Check sheet for the modelled part. Datum: model origin and axes. Units: mm. Round coordinates to 2 decimals unless told otherwise and drop trailing zeros. Loops run counter-clockwise (first coordinate to the right, second up) from the corner with the lowest first, then second, coordinate; pieces in that order, holes last. Notation, with made-up numbers: (62.5, -1.5) -> (73.5, -1.5) arc R30 ccw to (73.5, 32.5) -> close; hole circle Ø5 at (47.25, -16.5). An arc over 180 degrees is marked (long way). Use one line per item in the form item = value. Start each with the question number.
(1) Draft check along X on faces 1 (the cylindrical face through (74.1, -12.3, 45.4)), 2 (the cylindrical face through (76.7, -12.3, 40.1)), 3 (the flat face through (83, -25, 38)). Enter one of: released by +X, released by -X, zero draft, split by the parting line, or undercut.
(2) Sectioned sample at A-A (z = 40). Record the cut outline in (x, y).
(3) Go/stop test with flat-tipped pins: pin 1 (1 mm diameter, centred on y = -10, z = 41.5, fed in from +X); pin 2 (2 mm diameter, centred on y = -11, z = 36, fed in from -X); pin 3 (1.5 mm diameter, centred on x = 84.5, y = -14.5, fed in from +Z). Record where each tip stops, or that it passes through.
(4) Material ranges on probe 1 along Z at (x, y) = (80, -12.5); probe 2 along X at (y, z) = (-4.75, 37.25); probe 3 along X at (y, z) = (-13, 39.25), recorded low to high. Write a range as [from, to].
(5) Sectioned sample at C-C (y = -22.75). Record the cut outline in (x, z), and give its area (3 significant figures).
(6) Sectioned sample at B-B (x = 80.25). Record the cut outline in (y, z).
(7) Sectioned sample at D-D (x = 74.75). Record the cut outline in (y, z).
from build123d import *

# Parameters (mm, degrees)
CYLINDER011_R     = 3.3
CYLINDER011_DEPTH = 25
CYLINDER009_R     = 8
CYLINDER009_DEPTH = 25


with BuildPart() as zylinder011:
    # Cylinder011 → Cylinder011 (new body)
    with BuildSketch(Plane(origin=(80, 0, 40), x_dir=(1, 0, 0), z_dir=(0, -1, 0))):
        Circle(CYLINDER011_R)
    extrude(amount=CYLINDER011_DEPTH)


with BuildPart() as spacer01:
    # Cylinder009 → Cylinder009 (new body)
    with BuildSketch(Plane(origin=(80, 0, 40), x_dir=(1, 0, 0), z_dir=(0, -1, 0))):
        Circle(CYLINDER009_R)
    extrude(amount=CYLINDER009_DEPTH)

    # Cut006: cut Zylinder011
    add(zylinder011.part, mode=Mode.SUBTRACT)


solid = spacer01.part
Checks:
q1.face_1 = split by the parting line
q1.face_2 = undercut
q1.face_3 = zero draft
q2.outline = (72, -25) -> (76.7, -25) -> (76.7, 0) -> (72, 0) -> close; (83.3, -25) -> (88, -25) -> (88, 0) -> (83.3, 0) -> close
q3.pin_1 = 87.94
q3.pin_2 = 72.58
q3.pin_3 = 47.07
q4.probe_1 = [32, 36.7], [43.3, 48]
q4.probe_2 = [72.49, 78.18], [81.82, 87.51]
q4.probe_3 = [72.04, 76.79], [83.21, 87.96]
q5.outline = circle Ø16 at (80, 40); hole circle Ø6.6 at (80, 40)
q5.area = 167 mm2
q6.outline = (-25, 32) -> (0, 32) -> (0, 36.71) -> (-25, 36.71) -> close; (-25, 43.29) -> (0, 43.29) -> (0, 48) -> (-25, 48) -> close
q7.outline = (-25, 33.96) -> (0, 33.96) -> (0, 46.04) -> (-25, 46.04) -> close
